```python
from build123d import *

# Parameters (mm, degrees)
SKETCH_1_R          = 38
EXTRUDE_1_DEPTH     = 18
CUT_EXTRUDE_1_REACH = 20
SKETCH_2_R          = 1.5
CUT_EXTRUDE_2_DEPTH = 12.5
FILLET_1_R          = 1
CUT_EXTRUDE_7_REACH = 13
SKETCH_6_W          = 20
SKETCH_6_H          = 4
CUT_EXTRUDE_8_REACH = 20
SKETCH_7_R          = 2


with BuildPart() as part:
    # Эскиз1 → Бобышка-Вытянуть1 (new body)
    with BuildSketch(Plane.XY):
        Circle(SKETCH_1_R)
    extrude(amount=EXTRUDE_1_DEPTH)

    # Эскиз2 → Вырез-Вытянуть1 (cut, up to next)
    with BuildSketch(Plane.XY.offset(18), mode=Mode.PRIVATE) as cut_extrude_1_sk1:
        with Locations((-34, 0)):
            Circle(SKETCH_2_R)
    cut_extrude_1_tool1 = extrude(cut_extrude_1_sk1.sketch, amount=-CUT_EXTRUDE_1_REACH, mode=Mode.PRIVATE) & part.part
    add(cut_extrude_1_tool1.solids().sort_by_distance((-34, 0, 18))[0], mode=Mode.SUBTRACT)
    # Эскиз2 → Вырез-Вытянуть1 (cut, up to next)
    with BuildSketch(Plane.XY.offset(18), mode=Mode.PRIVATE) as cut_extrude_1_sk2:
        with Locations((-17, 29.444863729)):
            Circle(SKETCH_2_R)
    cut_extrude_1_tool2 = extrude(cut_extrude_1_sk2.sketch, amount=-CUT_EXTRUDE_1_REACH, mode=Mode.PRIVATE) & part.part
    add(cut_extrude_1_tool2.solids().sort_by_distance((-17, 29.444864, 18))[0], mode=Mode.SUBTRACT)
    # Эскиз2 → Вырез-Вытянуть1 (cut, up to next)
    with BuildSketch(Plane.XY.offset(18), mode=Mode.PRIVATE) as cut_extrude_1_sk3:
        with Locations((17, 29.444863729)):
            Circle(SKETCH_2_R)
    cut_extrude_1_tool3 = extrude(cut_extrude_1_sk3.sketch, amount=-CUT_EXTRUDE_1_REACH, mode=Mode.PRIVATE) & part.part
    add(cut_extrude_1_tool3.solids().sort_by_distance((17, 29.444864, 18))[0], mode=Mode.SUBTRACT)
    # Эскиз2 → Вырез-Вытянуть1 (cut, up to next)
    with BuildSketch(Plane.XY.offset(18), mode=Mode.PRIVATE) as cut_extrude_1_sk4:
        with Locations((34, 0)):
            Circle(SKETCH_2_R)
    cut_extrude_1_tool4 = extrude(cut_extrude_1_sk4.sketch, amount=-CUT_EXTRUDE_1_REACH, mode=Mode.PRIVATE) & part.part
    add(cut_extrude_1_tool4.solids().sort_by_distance((34, 0, 18))[0], mode=Mode.SUBTRACT)
    # Эскиз2 → Вырез-Вытянуть1 (cut, up to next)
    with BuildSketch(Plane.XY.offset(18), mode=Mode.PRIVATE) as cut_extrude_1_sk5:
        with Locations((17, -29.444863729)):
            Circle(SKETCH_2_R)
    cut_extrude_1_tool5 = extrude(cut_extrude_1_sk5.sketch, amount=-CUT_EXTRUDE_1_REACH, mode=Mode.PRIVATE) & part.part
    add(cut_extrude_1_tool5.solids().sort_by_distance((17, -29.444864, 18))[0], mode=Mode.SUBTRACT)
    # Эскиз2 → Вырез-Вытянуть1 (cut, up to next)
    with BuildSketch(Plane.XY.offset(18), mode=Mode.PRIVATE) as cut_extrude_1_sk6:
        with Locations((-17, -29.444863729)):
            Circle(SKETCH_2_R)
    cut_extrude_1_tool6 = extrude(cut_extrude_1_sk6.sketch, amount=-CUT_EXTRUDE_1_REACH, mode=Mode.PRIVATE) & part.part
    add(cut_extrude_1_tool6.solids().sort_by_distance((-17, -29.444864, 18))[0], mode=Mode.SUBTRACT)

    # Эскиз3 → Вырез-Вытянуть2 (cut)
    with BuildSketch(Plane(origin=(0, 0, 0), x_dir=(-1, 0, 0), z_dir=(0, 0, -1))):
        with BuildLine():
            Line((-13.076696831, -27), (13.076696831, -27))
            ThreePointArc((13.076696831, -27), (0, 30), (-13.076696831, -27))
        make_face()
    extrude(amount=-CUT_EXTRUDE_2_DEPTH, mode=Mode.SUBTRACT)

    # Скругление1
    fillet_1_edges = [part.edges().sort_by_distance(p)[0] for p in [
        (-38, 0, 18),
    ]]
    fillet(fillet_1_edges, radius=FILLET_1_R)

    # Эскиз6 → Вырез-Вытянуть7 (cut, up to next)
    with BuildSketch(Plane(origin=(0, -27, 0), x_dir=(1, 0, 0), z_dir=(0, 1, 0)), mode=Mode.PRIVATE) as cut_extrude_7_sk1:
        with Locations((0, -10.5)):
            Rectangle(SKETCH_6_W, SKETCH_6_H)
    cut_extrude_7_tool1 = extrude(cut_extrude_7_sk1.sketch, amount=-CUT_EXTRUDE_7_REACH, mode=Mode.PRIVATE) & part.part
    add(cut_extrude_7_tool1.solids().sort_by_distance((0, -27, 10.5))[0], mode=Mode.SUBTRACT)

    # Эскиз7 → Вырез-Вытянуть8 (cut, up to next)
    with BuildSketch(Plane.XY.offset(18), mode=Mode.PRIVATE) as cut_extrude_8_sk1:
        with Locations((0, 15.5)):
            Circle(SKETCH_7_R)
    cut_extrude_8_tool1 = extrude(cut_extrude_8_sk1.sketch, amount=-CUT_EXTRUDE_8_REACH, mode=Mode.PRIVATE) & part.part
    add(cut_extrude_8_tool1.solids().sort_by_distance((0, 15.5, 18))[0], mode=Mode.SUBTRACT)
    # Эскиз7 → Вырез-Вытянуть8 (cut, up to next)
    with BuildSketch(Plane.XY.offset(18), mode=Mode.PRIVATE) as cut_extrude_8_sk2:
        with Locations((13.423393759, 7.75)):
            Circle(SKETCH_7_R)
    cut_extrude_8_tool2 = extrude(cut_extrude_8_sk2.sketch, amount=-CUT_EXTRUDE_8_REACH, mode=Mode.PRIVATE) & part.part
    add(cut_extrude_8_tool2.solids().sort_by_distance((13.423394, 7.75, 18))[0], mode=Mode.SUBTRACT)
    # Эскиз7 → Вырез-Вытянуть8 (cut, up to next)
    with BuildSketch(Plane.XY.offset(18), mode=Mode.PRIVATE) as cut_extrude_8_sk3:
        with Locations((13.423393759, -7.75)):
            Circle(SKETCH_7_R)
    cut_extrude_8_tool3 = extrude(cut_extrude_8_sk3.sketch, amount=-CUT_EXTRUDE_8_REACH, mode=Mode.PRIVATE) & part.part
    add(cut_extrude_8_tool3.solids().sort_by_distance((13.423394, -7.75, 18))[0], mode=Mode.SUBTRACT)
    # Эскиз7 → Вырез-Вытянуть8 (cut, up to next)
    with BuildSketch(Plane.XY.offset(18), mode=Mode.PRIVATE) as cut_extrude_8_sk4:
        with Locations((0, -15.5)):
            Circle(SKETCH_7_R)
    cut_extrude_8_tool4 = extrude(cut_extrude_8_sk4.sketch, amount=-CUT_EXTRUDE_8_REACH, mode=Mode.PRIVATE) & part.part
    add(cut_extrude_8_tool4.solids().sort_by_distance((0, -15.5, 18))[0], mode=Mode.SUBTRACT)
    # Эскиз7 → Вырез-Вытянуть8 (cut, up to next)
    with BuildSketch(Plane.XY.offset(18), mode=Mode.PRIVATE) as cut_extrude_8_sk5:
        with Locations((-13.423393759, -7.75)):
            Circle(SKETCH_7_R)
    cut_extrude_8_tool5 = extrude(cut_extrude_8_sk5.sketch, amount=-CUT_EXTRUDE_8_REACH, mode=Mode.PRIVATE) & part.part
    add(cut_extrude_8_tool5.solids().sort_by_distance((-13.423394, -7.75, 18))[0], mode=Mode.SUBTRACT)
    # Эскиз7 → Вырез-Вытянуть8 (cut, up to next)
    with BuildSketch(Plane.XY.offset(18), mode=Mode.PRIVATE) as cut_extrude_8_sk6:
        with Locations((-13.423393759, 7.75)):
            Circle(SKETCH_7_R)
    cut_extrude_8_tool6 = extrude(cut_extrude_8_sk6.sketch, amount=-CUT_EXTRUDE_8_REACH, mode=Mode.PRIVATE) & part.part
    add(cut_extrude_8_tool6.solids().sort_by_distance((-13.423394, 7.75, 18))[0], mode=Mode.SUBTRACT)


solid = part.part
```
CAD build for the part. Positions are in the model's coordinates, mm. A direction names the side the tool comes from. Coordinates: 2 decimals unless noted, no trailing zeros. Order: outer loops, then holes, each group sorted by start corner. A loop starts at its lowest first (then second) coordinate and runs counter-clockwise, first axis right, second up.
(1) Mould opens along Y. For faces 4 (the face through (10, -32, 11)), 5 (the face through (20.43, 32.04, 8.38)), 6 (the face through (-14.9, 9.1, 15.3)), 7 (the face through (0, -4, 12.5)) say: released by +Y, released by -Y, zero draft, split by the parting line, or undercut.
Solution:
face 4: zero draft
face 5: split by the parting line
face 6: undercut
face 7: undercut
(2) Saw through at A-A, the plane y = 0. Write the cut outline in (x, z).
Solution:
outline: (-38, 0) - (-35.5, 0) - (-35.5, 18) - (-37, 18) arc R1 ccw to (-38, 17) - close; (-32.5, 0) - (-30, 0) - (-30, 12.5) - (30, 12.5) - (30, 0) - (32.5, 0) - (32.5, 18) - (-32.5, 18) - close; (35.5, 0) - (38, 0) - (38, 17) arc R1 ccw to (37, 18) - (35.5, 18) - close
(3) Saw through at C-C, the plane x = 17. Count the separate pieces of the cut face and the enclosed holes in it, and give its area (3 significant figures).
Solution:
separate pieces: 3
enclosed holes: 0
area: 497 mm2
(4) Which spindle directions (+Z, -Z, +X, -X, +Y, -Y) get a long thin tool onto all of the face, cutting with end or side? Do faces 1 (the face through (0, -27, 5)), 2 (the face through (-10, -32, 11)), 3 (the face through (-0.26, 17.483, 15.288)). Say none if no direction does.
Solution:
face 1: -Z
face 2: -Y
face 3: +Z, -Z
(5) Drill centre lines: L1, parallel to Y at x = 0, z = 16.05; L2, parallel to X at y = -7, z = 14; L3, parallel to Y at x = 17, z = 13. Where is each one in solid material? Low to high.
Solution:
L1: y = -38 to -17.5, -13.5 to 13.5, 17.5 to 38
L2: x = -37.35 to -15.28, -11.57 to 11.57, 15.28 to 37.35
L3: y = -33.99 to -30.94, -27.94 to 27.94, 30.94 to 33.99
(6) Pin check, flat tips, straight feed: pin 1 Ø6.5 at (x, y) = (-13.42, 7.75) entering from -Z; pin 2 Ø1.2 at (y, z) = (-29.5, 10) entering from -X; pin 3 Ø3 at (x, z) = (7.5, 6.5) entering from -Y. Stop position of each tip, or through.
Solution:
pin 1: stops at z = 12.5
pin 2: stops at x = -24.67
pin 3: stops at y = -37.52
(7) Saw through at B-B, the plane z = 5.25. Write the cut outline in (x, y), and give its area (3 significant figures).
Solution:
outline: circle Ø76 at (0, 0); hole circle Ø3 at (-34, 0); hole circle Ø3 at (-17, -29.44); hole circle Ø3 at (-17, 29.44); hole (-13.08, -27) - (13.08, -27) arc R30 ccw (long way) to start; hole circle Ø3 at (17, -29.44); hole circle Ø3 at (17, 29.44); hole circle Ø3 at (34, 0)
area: 1,720 mm2
